Answer from the drawing. Dimensions are ordinates in mm from the lowest x, y and z of the part. Coordinates: 2 decimals unless noted, no trailing zeros. Loops run counter-clockwise (first coordinate to the right, second up) from the corner with the lowest first, then second, coordinate; pieces in that order, holes last. Notation, with made-up numbers: (2.5, -11) -> (32.5, -11) arc R9 cw to (32.5, 3) -> close; hole circle Ø7 at (18, 82). An arc over 180 degrees is marked (long way). Answer as CSV lines item,"result".
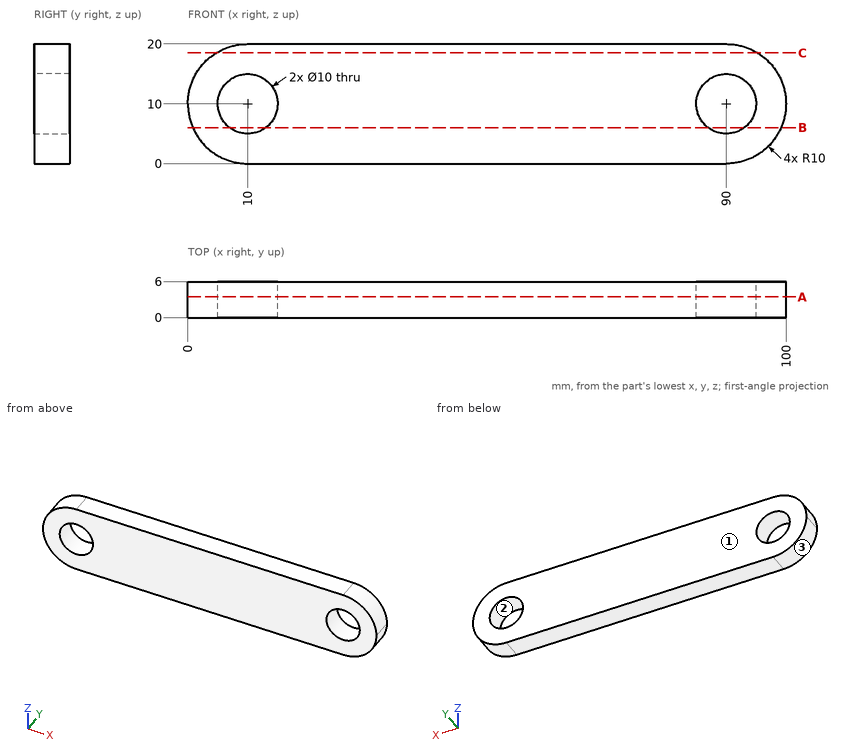
(1) A cutting plane is placed at A-A, the plane y = 3.45. Count the separate pieces of the cut face and the enclosed holes in it, and give its area (3 significant figures).
Computed values:
separate pieces,"1"
enclosed holes,"2"
area,"1,760 mm2"
(2) A cutting plane is placed at C-C, the plane z = 18.5. Write down the section's boundary in (x, y).
Computed values:
outline,"(4.73, 0) -> (95.27, 0) -> (95.27, 6) -> (4.73, 6) -> close"
(3) For a pull along X with two mould halves and no side action, classify the marked faces 1, 2 and 3 as pulls with the +X half, pulls with the -X half, needs draft (parallel to the pull), parting line crosses it, or undercut.
Computed values:
face 1,"needs draft"
face 2,"undercut"
face 3,"pulls with the -X half"
(4) Consider line 1 along X through (y, z) = (3.6, 10); line 2 along X through (y, z) = (0.35, 11.5); line 3 along X through (y, z) = (4.85, 18.75). Determine where each line is inside the solid, lowest interval first.
Computed values:
line 1,"0 to 5, 15 to 85, 95 to 100"
line 2,"0.11 to 5.23, 14.77 to 85.23, 94.77 to 99.89"
line 3,"5.16 to 94.84"
(5) A cutting plane is placed at B-B, the plane z = 6. Write down the section's boundary in (x, y) (3 decimals), and give its area (3 significant figures).
Computed values:
outline,"(0.835, 0) -> (7, 0) -> (7, 6) -> (0.835, 6) -> close; (13, 0) -> (87, 0) -> (87, 6) -> (13, 6) -> close; (93, 0) -> (99.165, 0) -> (99.165, 6) -> (93, 6) -> close"
area,"518 mm2"
(6) A flat-ended cylindrical pin translates along its axis: pin 1 Ø1 at (y, z) = (4.5, 13) entering from -X. Find the tip coordinate at first contact, or state that the pin passes through.
Computed values:
pin 1,"x = 0.32"
